Answer from the drawing. Dimensions are ordinates in mm from the lowest x, y and z of the part. Coordinates: 2 decimals unless noted, no trailing zeros. Write each loop counter-clockwise with the first axis right and the second up, starting at its lowest first coordinate (ties: lowest second). Pieces come first, ordered by that corner, then holes. Notation, with made-up numbers: (14.5, -37.75) - (22.5, -37.75) arc R36 ccw to (22.5, -3.75) - close; hole circle Ø5 at (15.25, 22.5). An arc over 180 degrees is marked (long way). Use one line per item in the form item = value. Start each with the question number.
Item 1: A cutting plane is placed at B-B (x = 97.5). Write down the section's boundary in (y, z), then the cut area to 3 significant figures.
Item 2: A cutting plane is placed at C-C (y = 2.75). Give the number of separate pieces and of enclosed holes in the cut face, then the cut area to 3 significant figures.
Item 3: A cutting plane is placed at D-D (z = 118). Write down the section's boundary in (x, y).
Item 4: A cutting plane is placed at A-A (z = 65). Write down the section's boundary in (x, y).
Item 5: Consider probe 1 along Z at (x, y) = (65, 2.5); probe 2 along X at (y, z) = (3.5, 81.5); probe 3 along X at (y, z) = (3.25, 94.5). Determine where each line is inside the solid, lowest interval first.
Item 6: Given pin 1 (1 mm diameter, centred on x = 47.5, z = 51.5, fed in from -Y), flat-ended and moving along its own axis, determine where the tip first touches the part or whether it passes through.
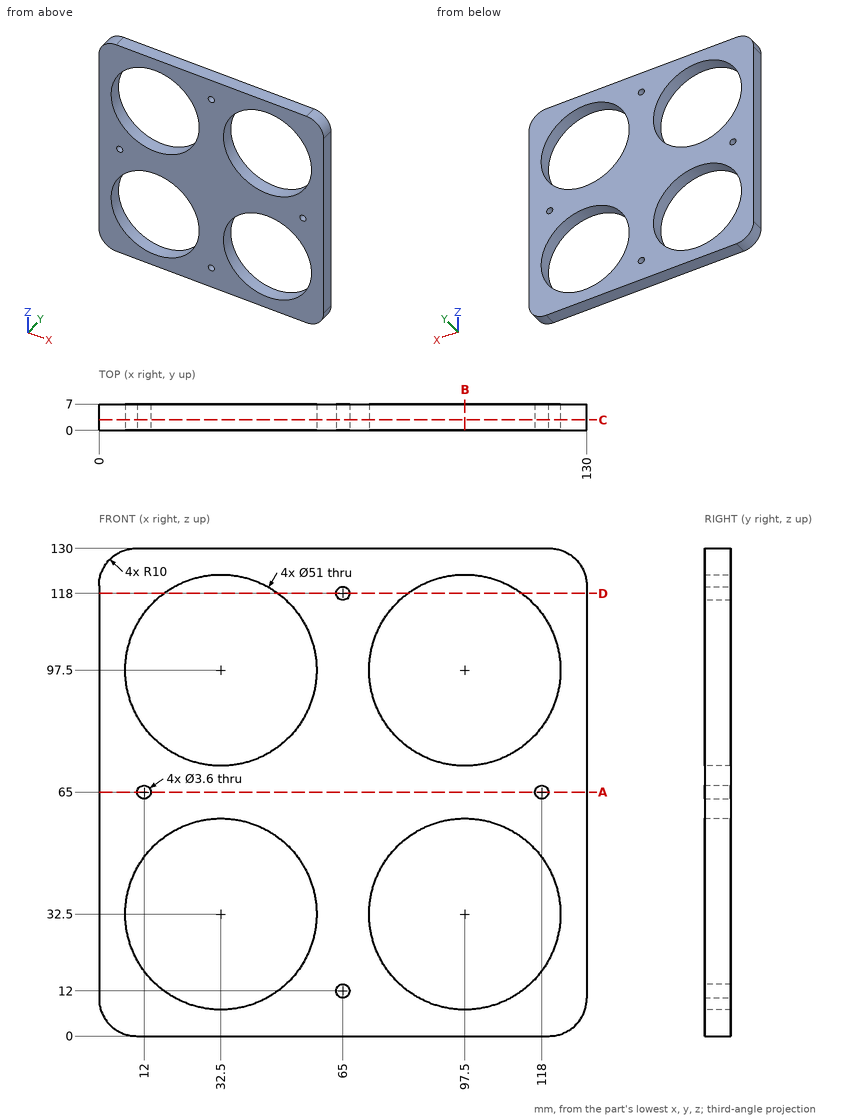
Answer:
q1.outline = (0, 0) - (7, 0) - (7, 7) - (0, 7) - close; (0, 58) - (7, 58) - (7, 72) - (0, 72) - close; (0, 123) - (7, 123) - (7, 130) - (0, 130) - close
q1.area = 196 mm²
q2.separate_pieces = 1
q2.enclosed_holes = 8
q2.area = 8,600 mm²
q3.outline = (0, 0) - (17.33, 0) - (17.33, 7) - (0, 7) - close; (47.67, 0) - (63.2, 0) - (63.2, 7) - (47.67, 7) - close; (66.8, 0) - (82.33, 0) - (82.33, 7) - (66.8, 7) - close; (112.67, 0) - (130, 0) - (130, 7) - (112.67, 7) - close
q4.outline = (0, 0) - (10.2, 0) - (10.2, 7) - (0, 7) - close; (13.8, 0) - (116.2, 0) - (116.2, 7) - (13.8, 7) - close; (119.8, 0) - (130, 0) - (130, 7) - (119.8, 7) - close
q5.probe_1 = 0 to 10.2, 13.8 to 116.2, 119.8 to 130
q5.probe_2 = 0 to 12.64, 52.36 to 77.64, 117.36 to 130
q5.probe_3 = 0 to 7.18, 57.82 to 72.18, 122.82 to 130
q6.pin_1 = through
